```python
from build123d import *

# Parameters (mm, degrees)
BOSS_EXTRUDE1_DEPTH = 110
CUT_EXTRUDE1_DEPTH  = 109.5
SKETCH3_R           = 2.875
CUT_EXTRUDE2_DEPTH  = 5


with BuildPart() as part:
    # Sketch1 → Boss-Extrude1 (new body)
    with BuildSketch(Plane(origin=(0, 0, 0), x_dir=(1, 0, 0), z_dir=(0, 1, 0))):
        with BuildLine():
            Line((-43.883093525, -1.707733813), (1.116906475, -1.707733813))
            Line((1.116906475, -1.707733813), (1.116906475, 18.292266187))
            ThreePointArc((1.116906475, 18.292266187), (-21.383093525, 40.792266187), (-43.883093525, 18.292266187))
            Line((-43.883093525, 18.292266187), (-43.883093525, -1.707733813))
        make_face()
    extrude(amount=BOSS_EXTRUDE1_DEPTH)

    # Sketch2 → Cut-Extrude1 (cut)
    with BuildSketch(Plane(origin=(0, 110, 0), x_dir=(1, 0, 0), z_dir=(0, 1, 0))):
        with BuildLine():
            Line((-43.383093525, 16.292266187), (-43.383093525, 13.292266187))
            Line((-43.383093525, 13.292266187), (-39.383093525, 13.292266187))
            Line((-39.383093525, 13.292266187), (-39.383093525, 11.292266187))
            Line((-39.383093525, 11.292266187), (-43.383093525, 11.292266187))
            Line((-43.383093525, 11.292266187), (-43.383093525, -1.207733813))
            Line((-43.383093525, -1.207733813), (0.616906475, -1.207733813))
            Line((0.616906475, -1.207733813), (0.616906475, 11.292266187))
            Line((0.616906475, 11.292266187), (-3.383093525, 11.292266187))
            Line((-3.383093525, 11.292266187), (-3.383093525, 13.292266187))
            Line((-3.383093525, 13.292266187), (0.616906475, 13.292266187))
            Line((0.616906475, 13.292266187), (0.616906475, 16.292266187))
            Line((0.616906475, 16.292266187), (-3.383093525, 16.292266187))
            Line((-3.383093525, 16.292266187), (-3.383093525, 18.292266187))
            Line((-3.383093525, 18.292266187), (0.616906475, 18.292266187))
            ThreePointArc((0.616906475, 18.292266187), (-21.383093525, 40.292266187), (-43.383093525, 18.292266187))
            Line((-43.383093525, 18.292266187), (-39.383093525, 18.292266187))
            Line((-39.383093525, 18.292266187), (-39.383093525, 16.292266187))
            Line((-39.383093525, 16.292266187), (-43.383093525, 16.292266187))
        make_face()
    extrude(amount=-CUT_EXTRUDE1_DEPTH, mode=Mode.SUBTRACT)

    # Sketch3 → Cut-Extrude2 (cut)
    with BuildSketch(Plane.ZY.offset(43.883093525)):
        with Locations((-4.958932854, 55)):
            Circle(SKETCH3_R)
    extrude(amount=-CUT_EXTRUDE2_DEPTH, mode=Mode.SUBTRACT)


solid = part.part
```
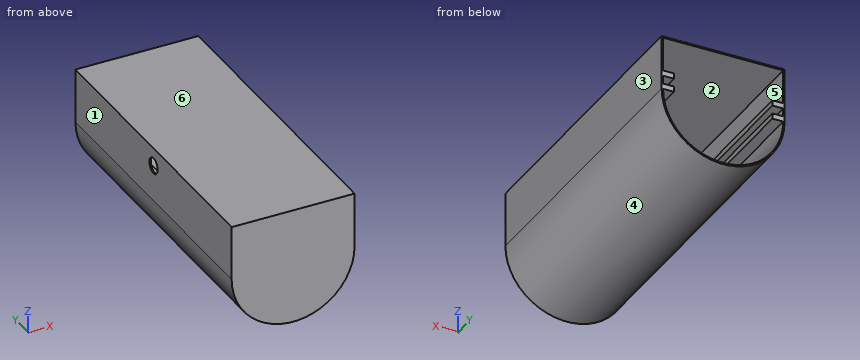
Model file for the job. Use its own axes, mm. Face numbers are marked on the shaded views. A direction names the side the tool comes from. Round coordinates to 2 decimals unless told otherwise and drop trailing zeros. Write each loop counter-clockwise with the first axis right and the second up, starting at its lowest first coordinate (ties: lowest second). Pieces come first, ordered by that corner, then holes. Notation, with made-up numbers: (70.25, 87.5) - (123.25, 87.5) arc R13 ccw to (123.25, 103.5) - close; hole circle Ø10 at (-24.75, 52). An arc over 180 degrees is marked (long way). Use CSV: the item, a comma, the result in double quotes. Start each with the question number.
Item 1: Drill centre lines: L1, parallel to X at y = 91.5, z = -17; L2, parallel to Z at x = -2.5, y = 24.5; L3, parallel to Y at x = -23, z = -38. Where is each one in solid material? Low to high. Write a range as [from, to].
Item 2: Band-saw the part on A-A (y = 32). Write the cut outline in (x, z), and give its area (3 significant figures).
Item 3: Band-saw the part on D-D (z = -20). Write the cut outline in (x, y), and give its area (3 significant figures).
Item 4: Pin check, flat tips, straight feed: P1, Ø1.5, axis at x = -7, z = -9, coming from the +Y side; P2, Ø1.5, axis at y = 79.5, z = -27, coming from the +X side; P3, Ø2, axis at x = -0.5, y = 79, coming from the -Z side. Stop position of each tip, or through.
Item 5: Tool access for the marked faces 1 and 2: list every direction of +Z, -Z, +X, -X, +Y, -Y with a clear straight run to the whole face (end or side of a thin tool).
Item 6: Band-saw the part on C-C (x = -14.5). Write the cut outline in (y, z).
Item 7: Two-plate mould, pull along Z, no slides. Class the marked faces 3, 4, 5 and 6: released by +Z, released by -Z, zero draft, split by the parting line, or undercut.
Item 8: Band-saw the part on B-B (y = 55). Write the cut outline in (x, z), and give its area (3 significant figures).
Checked values:
1,L1,"x = [-43.88, -39.38], [-3.38, 1.12]"
1,L2,"z = [-30.53, -29.58], [-18.29, -16.29], [-13.29, -11.29], [1.21, 1.71]"
1,L3,"y = [0, 0.5]"
2,outline,"(-43.88, -18.29) arc R22.5 ccw to (1.12, -18.29) - (1.12, 1.71) - (-43.88, 1.71) - close; hole (-43.38, -18.29) arc R22 ccw to (0.62, -18.29) - (-3.38, -18.29) - (-3.38, -16.29) - (0.62, -16.29) - (0.62, -13.29) - (-3.38, -13.29) - (-3.38, -11.29) - (0.62, -11.29) - (0.62, 1.21) - (-43.38, 1.21) - (-43.38, -11.29) - (-39.38, -11.29) - (-39.38, -13.29) - (-43.38, -13.29) - (-43.38, -16.29) - (-39.38, -16.29) - (-39.38, -18.29) - close"
2,area,"109 mm²"
3,outline,"(-43.82, 0) - (1.05, 0) - (1.05, 110) - (0.55, 110) - (0.55, 0.5) - (-43.32, 0.5) - (-43.32, 110) - (-43.82, 110) - close"
3,area,"132 mm²"
4,P1,"stops at y = 0.5"
4,P2,"stops at x = -0.34"
4,P3,"stops at z = -28.82"
5,face 1,"+Z, -Z, -X, +Y, -Y"
5,face 2,"+Y"
6,outline,"(0, -39.71) - (110, -39.71) - (110, -39.19) - (0.5, -39.19) - (0.5, 1.21) - (110, 1.21) - (110, 1.71) - (0, 1.71) - close"
7,face 3,"zero draft"
7,face 4,"released by -Z"
7,face 5,"undercut"
7,face 6,"released by +Z"
8,outline,"(-43.88, -18.29) arc R22.5 ccw to (1.12, -18.29) - (1.12, 1.71) - (-43.88, 1.71) - (-43.88, -2.08) - (-43.38, -2.08) - (-43.38, 1.21) - (0.62, 1.21) - (0.62, -11.29) - (-3.38, -11.29) - (-3.38, -13.29) - (0.62, -13.29) - (0.62, -16.29) - (-3.38, -16.29) - (-3.38, -18.29) - (0.62, -18.29) arc R22 cw to (-43.38, -18.29) - (-39.38, -18.29) - (-39.38, -16.29) - (-43.38, -16.29) - (-43.38, -13.29) - (-39.38, -13.29) - (-39.38, -11.29) - (-43.38, -11.29) - (-43.38, -7.83) - (-43.88, -7.83) - close"
8,area,"106 mm²"
